Source: CAD feature listing. Evaluate the final solid. Frame: model axes, mm. A direction names the side the tool comes from. Give positions to 0.01 mm unless a question says otherwise; leave off trailing zeros. Write each loop counter-clockwise with the first axis right and the second up, starting at its lowest first coordinate (ties: lowest second). Pieces come first, ordered by that corner, then holes. Notation, with made-up numbers: (41, -5) -> (73, -5) arc R18 ccw to (73, 16) -> close; hole circle Ø10 at (-20, 87.25). An arc over 180 degrees is marked (long way). Answer as a JSON object with one key per item and string values. Group by question number.
Item 1: Ray query, probe 1 along Z at (x, y) = (-37.5, 5.75); probe 2 along Z at (x, y) = (-48.5, 1.75); probe 3 along X at (y, z) = (1.5, 80). Return the intervals inside material, ascending. Write a range as from..to.
Item 2: Section query A-A on x = -48.5. Return the cut outline in (y, z), plus the area to 3 significant figures.
Item 3: Section query C-C on z = 9. Return the cut outline in (x, y).
Item 4: Section query B-B on z = 70.5. Return the cut outline in (x, y), plus the area to 3 significant figures.
Item 5: Access query for faces 4 (the face through (-24, 3, 78.202)), 5 (the face through (-24.72, 2.958, 50.103)), 6 (the face through (-21.9, 3.09, 15.99)). Directions: +Z, -Z, +X, -X, +Y, -Y. A direction counts if a zero-diameter tool reaches every point of the face in a straight line with its end or side. Return the directions, or none.
Item 6: Section query D-D on z = 43.5. Return the cut outline in (x, y), plus the area to 3 significant figures.
Item 7: First-contact query: pin 1 Ø1.8 at (y, z) = (2.5, 33.5) entering from -X; pin 2 Ø2.5 at (x, y) = (-24, 3) entering from -Z; pin 3 Ø1.3 at (x, y) = (-23, 3.5) entering from +Z. Flat tips, straight axial feed; report the tip coordinate or a pass-through.
Item 8: Pull-direction query (Y, two-part tool) for faces 1 (the face through (-36, 0, 49)), 2 (the face through (-38, 3, 96.202)), 3 (the face through (-54, 3, 78.202)); classes: pulls with the +Y half, pulls with the -Y half, needs draft (parallel to the pull), parting line crosses it, or undercut.
from build123d import *

# Parameters (mm, degrees)
SKETCH1_W                     = 78
SKETCH1_H                     = 96.2019
BOSS_EXTRUDE1_DEPTH           = 6
SKETCH2_R                     = 1.5
CUT_EXTRUDE2_DEPTH            = 124.995183631
SKETCH3_R                     = 2.1
CUT_EXTRUDE3_DEPTH            = 18
CUT_EXTRUDE4_START            = -78.2019
SKETCH3_2_R                   = 2.1
CUT_EXTRUDE4_DEPTH            = 18
FILLET1_R                     = 5
CUT_EXTRUDE5_DEPTH            = 10
CSK_FOR_M3_SFHCS2_D           = 3.4
CSK_FOR_M3_SFHCS2_CSINK_D     = 7.12
CSK_FOR_M3_SFHCS2_CSINK_ANGLE = 90


with BuildPart() as part:
    # Sketch1 → Boss-Extrude1 (new body)
    with BuildSketch(Plane(origin=(0, 0, 0), x_dir=(-1, 0, 0), z_dir=(0, 1, 0))):
        with Locations((39, 48.10095)):
            Rectangle(SKETCH1_W, SKETCH1_H)
    extrude(amount=BOSS_EXTRUDE1_DEPTH)

    # Sketch2 → Cut-Extrude2 (cut, through all)
    with BuildSketch(Plane(origin=(0, 0, 0), x_dir=(-1, 0, 0), z_dir=(0, -1, 0))):
        with Locations(Location((75, -31.10095, 0), (0, 0, 90))):
            Circle(SKETCH2_R)
        with Locations(Location((75, -65.10095, 0), (0, 0, 90))):
            Circle(SKETCH2_R)
    extrude(amount=-CUT_EXTRUDE2_DEPTH, mode=Mode.SUBTRACT)

    # Sketch3 → Cut-Extrude3 (cut)
    with BuildSketch(Plane(origin=(0, 0, 0), x_dir=(1, 0, 0), z_dir=(0, 0, -1))):
        with Locations(Location((-54, -3, 0), (0, 0, 180))):
            Circle(SKETCH3_R)
        with Locations(Location((-24, -3, 0), (0, 0, 180))):
            Circle(SKETCH3_R)
    extrude(amount=-CUT_EXTRUDE3_DEPTH, mode=Mode.SUBTRACT)

    # Sketch3<2> → Cut-Extrude4 (cut)
    with BuildSketch(Plane(origin=(0, 0, 0), x_dir=(1, 0, 0), z_dir=(0, 0, -1)).offset(CUT_EXTRUDE4_START)):
        with Locations(Location((-54, -3, 0), (0, 0, 180))):
            Circle(SKETCH3_2_R)
        with Locations(Location((-24, -3, 0), (0, 0, 180))):
            Circle(SKETCH3_2_R)
    extrude(amount=-CUT_EXTRUDE4_DEPTH, mode=Mode.SUBTRACT)

    # Fillet1
    # the kernel refuses this fillet: 5 mm, written as the material it takes off along each edge
    with BuildSketch(Plane(origin=(-78, 0, -12.5), x_dir=(1, 0, 0), z_dir=(0, 0, 1))) as fillet1_piece_1:
        with BuildLine():
            CenterArc((FILLET1_R, FILLET1_R), FILLET1_R, 180, 90)
            Line((0, FILLET1_R), (0, 0))
            Line((0, 0), (FILLET1_R, 0))
        make_face()
    extrude(amount=121.2019, mode=Mode.SUBTRACT)

    # Sketch4 → Cut-Extrude5 (cut)
    with BuildSketch(Plane.XZ):
        with BuildLine():
            Line((-51, 92.2019), (-25, 92.2019))
            ThreePointArc((-25, 92.2019), (-20, 87.2019), (-25, 82.2019))
            Line((-25, 82.2019), (-51, 82.2019))
            ThreePointArc((-51, 82.2019), (-56, 87.2019), (-51, 92.2019))
        make_face()
        with BuildLine():
            Line((-58.5, 29.10095), (-58.5, 36.10095))
            ThreePointArc((-58.5, 36.10095), (-48.5, 46.10095), (-38.5, 36.10095))
            Line((-38.5, 36.10095), (-38.5, 29.10095))
            ThreePointArc((-38.5, 29.10095), (-48.5, 19.10095), (-58.5, 29.10095))
        make_face()
        with BuildLine():
            Line((-38.5, 67.10095), (-38.5, 60.10095))
            ThreePointArc((-38.5, 60.10095), (-48.5, 50.10095), (-58.5, 60.10095))
            Line((-58.5, 60.10095), (-58.5, 67.10095))
            ThreePointArc((-58.5, 67.10095), (-48.5, 77.10095), (-38.5, 67.10095))
        make_face()
        with BuildLine():
            Line((-14.5, 29.10095), (-14.5, 36.10095))
            ThreePointArc((-14.5, 36.10095), (-24.5, 46.10095), (-34.5, 36.10095))
            Line((-34.5, 36.10095), (-34.5, 29.10095))
            ThreePointArc((-34.5, 29.10095), (-24.5, 19.10095), (-14.5, 29.10095))
        make_face()
        with BuildLine():
            Line((-34.5, 67.10095), (-34.5, 60.10095))
            ThreePointArc((-34.5, 60.10095), (-24.5, 50.10095), (-14.5, 60.10095))
            Line((-14.5, 60.10095), (-14.5, 67.10095))
            ThreePointArc((-14.5, 67.10095), (-24.5, 77.10095), (-34.5, 67.10095))
        make_face()
        with BuildLine():
            Line((-51, 4), (-25, 4))
            ThreePointArc((-25, 4), (-20, 9), (-25, 14))
            Line((-25, 14), (-51, 14))
            ThreePointArc((-51, 14), (-56, 9), (-51, 4))
        make_face()
    extrude(amount=-CUT_EXTRUDE5_DEPTH, mode=Mode.SUBTRACT)

    # CSK for M3 SFHCS2 (through all)
    with Locations(Plane(origin=(0, 0, 0), x_dir=(-1, 0, 0), z_dir=(0, -1, 0))):
        with Locations((75, -31.10095), (75, -65.10095)):
            CounterSinkHole(CSK_FOR_M3_SFHCS2_D / 2, CSK_FOR_M3_SFHCS2_CSINK_D / 2, counter_sink_angle=CSK_FOR_M3_SFHCS2_CSINK_ANGLE)


solid = part.part
Worked answers:
{
 "1": {"probe 1": "0..4, 14..82.2, 92.2..96.2", "probe 2": "0..4, 14..19.1, 46.1..50.1, 77.1..82.2, 92.2..96.2", "probe 3": "-76.57..-55.47, -52.53..-25.47, -22.53..0"},
 "2": {"outline": "(0, 0) -> (6, 0) -> (6, 4) -> (0, 4) -> close; (0, 14) -> (6, 14) -> (6, 19.1) -> (0, 19.1) -> close; (0, 46.1) -> (6, 46.1) -> (6, 50.1) -> (0, 50.1) -> close; (0, 77.1) -> (6, 77.1) -> (6, 82.2) -> (0, 82.2) -> close; (0, 92.2) -> (6, 92.2) -> (6, 96.2) -> (0, 96.2) -> close", "area": "133 mm^2"},
 "3": {"outline": "(-78, 5) arc R5 ccw to (-73, 0) -> (-56, 0) -> (-56, 2.36) arc R2.1 cw to (-56, 3.64) -> (-56, 6) -> (-78, 6) -> close; (-20, 0) -> (0, 0) -> (0, 6) -> (-20, 6) -> close"},
 "4": {"outline": "(-78, 5) arc R5 ccw to (-73, 0) -> (-57.9, 0) -> (-57.9, 6) -> (-78, 6) -> close; (-39.1, 0) -> (-33.9, 0) -> (-33.9, 6) -> (-39.1, 6) -> close; (-15.1, 0) -> (0, 0) -> (0, 6) -> (-15.1, 6) -> close", "area": "237 mm^2"},
 "5": {"face 4": "+Z", "face 5": "+Y, -Y", "face 6": "-Z"},
 "6": {"outline": "(-78, 5) arc R5 ccw to (-73, 0) -> (-55.23, 0) -> (-55.23, 6) -> (-78, 6) -> close; (-41.77, 0) -> (-31.23, 0) -> (-31.23, 6) -> (-41.77, 6) -> close; (-17.77, 0) -> (0, 0) -> (0, 6) -> (-17.77, 6) -> close", "area": "301 mm^2"},
 "7": {"pin 1": "x = -77.74", "pin 2": "z = 18", "pin 3": "z = 78.2"},
 "8": {"face 1": "pulls with the -Y half", "face 2": "needs draft", "face 3": "undercut"}
}
